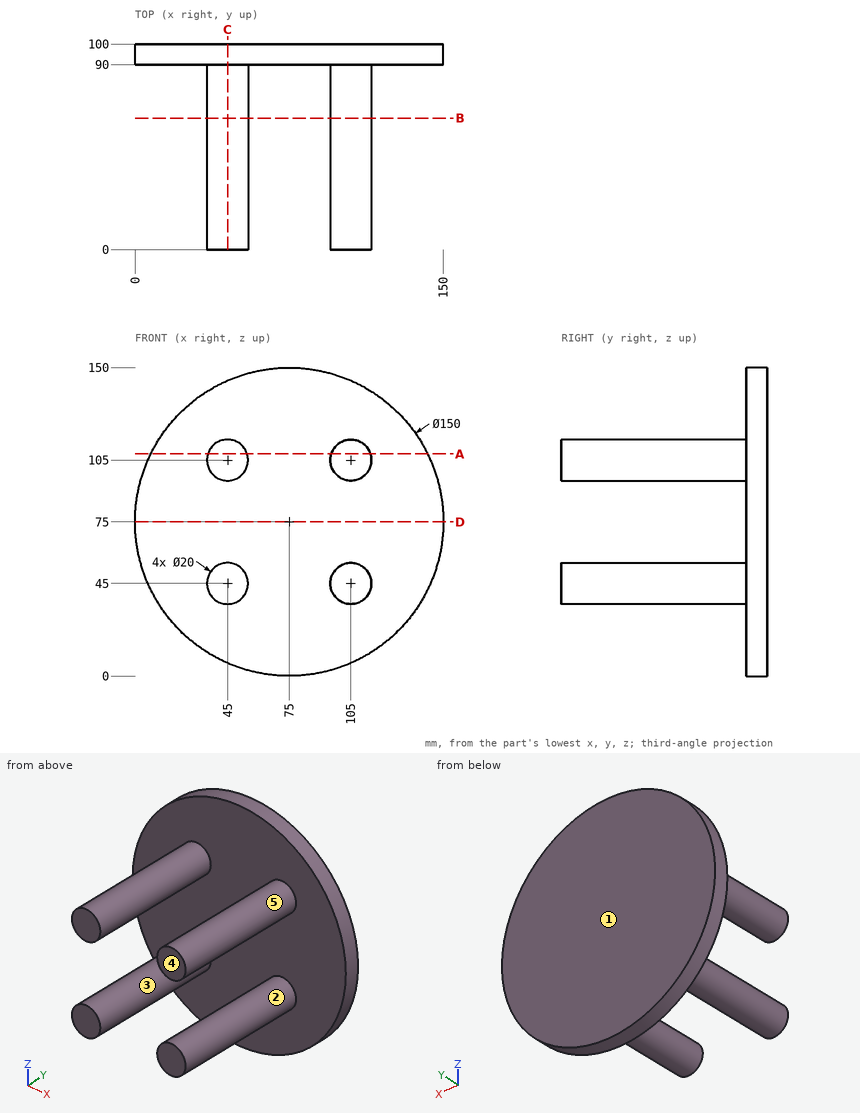
Print and shaded views of the part. All mm, measured from the part's lowest x, y and z. A direction names the side the tool comes from. Coordinates: 2 decimals unless noted, no trailing zeros. Loops run counter-clockwise (first coordinate to the right, second up) from the corner with the lowest first, then second, coordinate; pieces in that order, holes last. Notation, with made-up numbers: M 43.5,19.25 L 61.5,19.25 A25 ccw 61.5,52.25 Z; hole C 63.25,49 d7. An arc over 180 degrees is marked long. Use a Markdown table: item, result. Add a question column.
Q1. Cut at D-D (z = 75). Write the cut outline in (x, y).
Q2. Which spindle directions (+Z, -Z, +X, -X, +Y, -Y) get a long thin tool onto all of the face, cutting with end or side? Do the marked faces 4 and 5. Say none if no direction does.
Q3. Cut at C-C (x = 45). Write the cut outline in (y, z), and give its area (3 significant figures).
Q4. Cut at A-A (z = 108). Write the cut outline in (x, y).
Q5. Cut at B-B (y = 64). Write the cut outline in (x, z).
Q6. Mould opens along X. For the marked faces 1, 2 and 3 say: +X half, -X half, draft (parallel to the pull), parting line (faces both ways), or undercut.
Q7. Pin check, flat tips, straight feed: P1, Ø12, axis at x = 93.5, y = 16, coming from the -Z side; P2, Ø5, axis at x = 17.5, z = 26.5, coming from the -Y side; P3, Ø1, axis at y = 19.5, z = 47.5, coming from the -X side; P4, Ø12, axis at y = 31.5, z = 125.5, coming from the -X side. Stop position of each tip, or through.
Q8. Probe L1, parallel to X at y = 63, z = 45; L2, parallel to Y at x = 18.5, z = 36; L3, parallel to Z at x = 101, y = 6. List the from-to ranges inside material, lowest first.
Worked out:
| question | item | result |
|---|---|---|
| 1 | outline | M 0,90 L 150,90 L 150,100 L 0,100 Z |
| 2 | face 4 | +Z, -Z, +X, -X, -Y |
| 2 | face 5 | -Y |
| 3 | outline | M 0,35 L 90,35 L 90,6.26 L 100,6.26 L 100,143.74 L 90,143.74 L 90,115 L 0,115 L 0,95 L 90,95 L 90,55 L 0,55 Z |
| 3 | area | 4,970 mm2 |
| 4 | outline | M 7.65,90 L 35.46,90 L 35.46,0 L 54.54,0 L 54.54,90 L 95.46,90 L 95.46,0 L 114.54,0 L 114.54,90 L 142.35,90 L 142.35,100 L 7.65,100 Z |
| 5 | outline | C 45,45 d20; C 45,105 d20; C 105,45 d20; C 105,105 d20 |
| 6 | face 1 | draft |
| 6 | face 2 | undercut |
| 6 | face 3 | undercut |
| 7 | P1 | stops at z = 36.65 |
| 7 | P2 | stops at y = 90 |
| 7 | P3 | stops at x = 35.2 |
| 7 | P4 | passes through |
| 8 | L1 | x = 35 to 55, 95 to 115 |
| 8 | L2 | y = 90 to 100 |
| 8 | L3 | z = 35.83 to 54.17, 95.83 to 114.17 |
